Can you work these out from the model? Positions are in its coordinate system, mm. A direction names the side the tool comes from. Round coordinates to 2 decimals unless told otherwise and drop trailing zeros. Loops run counter-clockwise (first coordinate to the right, second up) from the corner with the lowest first, then second, coordinate; pieces in that order, holes last. Notation, with made-up numbers: M -7,-24 L 44,-24 A25 ccw 44,-11 Z; hole C 0.25,-24 d9. An arc over 180 degrees is marked long. Answer as CSV lines item,"result".
from build123d import *

# Parameters (mm, degrees)
F1_DEPTH       = 20
F2_R           = 1
F3_R           = 8
F5_D           = 4
F5_CSINK_D     = 7
F5_CSINK_ANGLE = 120


with BuildPart() as f1:
    # F0 (on Front) → F1 (new body)
    with BuildSketch(Plane.XZ):
        with BuildLine():
            Line((-16, 2), (-16, 0))
            Line((-16, 0), (16, 0))
            Line((16, 0), (16, 2))
            Line((16, 2), (8.8741196746, 2))
            ThreePointArc((8.8741196746, 2), (6.9647131351, 2.8862569391), (6.4090864317, 4.9166666667))
            ThreePointArc((6.4090864317, 4.9166666667), (5.8371497595, 8.8596647854), (3.0720549025, 11.7282177574))
            add(Edge.make_bspline(
                [(2.2805033402, 8.6550526389), (2.7656288893, 9.9644009916), (3.0720549025, 11.7282177574)],
                knots=[0.7096553764, 0.7096553764, 0.7096553764, 1.0711038861, 1.0711038861, 1.0711038861], degree=2, weights=[1, 0.9837137717, 1]))
            ThreePointArc((2.2805033402, 8.6550526389), (0, 2.5), (-2.2805033402, 8.6550526389))
            add(Edge.make_bspline(
                [(-3.0720549025, 11.7282177574), (-2.7656288893, 9.9644009916), (-2.2805033402, 8.6550526389)],
                knots=[5.2120814211, 5.2120814211, 5.2120814211, 5.5735299308, 5.5735299308, 5.5735299308], degree=2, weights=[1, 0.9837137717, 1]))
            ThreePointArc((-3.0720549025, 11.7282177574), (-5.8371497595, 8.8596647854), (-6.4090864317, 4.9166666667))
            ThreePointArc((-6.4090864317, 4.9166666667), (-6.9647131351, 2.8862569391), (-8.8741196746, 2))
            Line((-8.8741196746, 2), (-16, 2))
        make_face()
    extrude(amount=F1_DEPTH)

    # F2
    f2_edges = [f1.edges().sort_by_distance(p)[0] for p in [
        (-3.072055, -10, 11.728218),
        (3.072055, -10, 11.728218),
    ]]
    fillet(f2_edges, radius=F2_R)

    # F3
    f3_edges = [f1.edges().sort_by_distance(p)[0] for p in [
        (-16, -20, 1),
        (16, -20, 1),
        (16, 0, 1),
        (-16, 0, 1),
    ]]
    fillet(f3_edges, radius=F3_R)

    # F5 (through all)
    with Locations(Plane.XY.offset(2)):
        with Locations((-12.5, -10), (12.5, -10)):
            CounterSinkHole(F5_D / 2, F5_CSINK_D / 2, counter_sink_angle=F5_CSINK_ANGLE)


solid = f1.part
Item 1: Will these pins go through, and if not, where does the flat tip stop? pin 1 (2 mm diameter, centred on x = -13.5, y = -7.5, fed in from +Z); pin 2 (2 mm diameter, centred on y = -3, z = 2, fed in from -X); pin 3 (5.5 mm diameter, centred on x = 11, y = -9, fed in from +Z); pin 4 (6.5 mm diameter, centred on x = 0, z = 6, fed in from +Y).
Output:
pin 1,"stops at z = 2"
pin 2,"stops at x = -14.93"
pin 3,"stops at z = 2.08"
pin 4,"passes through"
Item 2: If we section it at D-D on x = -8.5: Write out the boundary of the cut face in (y, z).
Output:
outline,"M -19.98,0 L -0.02,0 L -0.02,2.03 L -19.98,2.03 Z"
Item 3: We'd pull the mould along X, two halves only. Please class faces 3 (the face through (-9.2, -7.6, 2)), 4 (the face through (13.974, -8.648, 0.559)), 5 (the face through (-16, -10, 1)): released by +X, released by -X, zero draft, split by the parting line, or undercut.
Output:
face 3,"zero draft"
face 4,"undercut"
face 5,"released by -X"
Item 4: On a 3-axis mill with a long thin cutter (end or side, diameter ignored), from which of +Z, -Z, +X, -X, +Y, -Y can I reach the whole of each face in a straight line? I mean faces 1 (the face through (9.3, -12.1, 2)), 2 (the face through (0, 0, 2)). Say none if no direction works.
Output:
face 1,"+Z, +X, +Y, -Y"
face 2,"+Z, -Z, +X, -X, +Y"
Item 5: If we section it at C-C on x = 0: Write out the boundary of the cut face in (y, z).
Output:
outline,"M -20,0 L 0,0 L 0,2.5 L -20,2.5 Z"
Item 6: If we section it at B-B on x = -12.5: Write out the boundary of the cut face in (y, z), then the cut area to 3 significant figures.
Output:
outline,"M -18.61,0 L -12,0 L -12,1.13 L -13.5,2 L -18.61,2 Z; M -8,0 L -1.39,0 L -1.39,2 L -6.5,2 L -8,1.13 Z"
area,"25.2 mm2"
Item 7: If I drill on line 1 along X through (y, z) = (-10, 0.5); line 2 along X through (y, z) = (-5.5, 6); line 3 along Z through (x, y) = (-15, -12.5), over which ranges is the centre line in solid material (lowest first)? Write a range as from..to.
Output:
line 1,"x = -16..-14.5, -10.5..10.5, 14.5..16"
line 2,"x = -6.5..-3.5, 3.5..6.5"
line 3,"z = 0..2"
Item 8: If we section it at A-A on z = 6: Write out the boundary of the cut face in (x, y).
Output:
outline,"M -6.5,-20 L -3.5,-20 L -3.5,0 L -6.5,0 Z; M 3.5,-20 L 6.5,-20 L 6.5,0 L 3.5,0 Z"
